Check sheet for the modelled part. Datum: model origin and axes. Units: mm. A direction names the side the tool comes from. Round coordinates to 2 decimals unless told otherwise and drop trailing zeros. Write each loop counter-clockwise with the first axis right and the second up, starting at its lowest first coordinate (ties: lowest second). Pieces come first, ordered by that corner, then holes. Notation, with made-up numbers: (66.5, 85.5) -> (109.5, 85.5) arc R20 cw to (109.5, 114.5) -> close; hole circle Ø8 at (35.5, 62.5). An arc over 180 degrees is marked (long way). Put each result on its own line as item: value. Start each with the question number.
Autodesk Inventor part; units mm, degrees
ref_plane "Work Plane2" through (-11, 0, 0) normal (1, 0, 0) x (0, 0, -1)
ref_plane "Work Plane3" through (0, 27, 0) normal (0, -1, 0) x (1, 0, 0)
ref_plane "YZ Plane" through (0, 0, 0) normal (1, 0, 0) x (0, 1, 0)
sketch "Sketch1" plane through (0, 0, 0) normal (0, 1, 0) x (-1, 0, 0)
  line L0 (0, 0) -> (22, 0)
  line L1 (22, 0) -> (22, -50)
  line L2 (22, -50) -> (0, -50)
  line L3 (0, -50) -> (0, 0)
  circle A0 centre (11, -8.5) radius 2.05
  circle A1 centre (11, -41.5) radius 2.05
  line L4 (22, 0) -> (0, -50) construction
  line L5 (22, -50) -> (0, 0) construction
  point P0 (11, -25)
  dimension "d0" = 22
  dimension "d1" = 50
  dimension "d2" = 4.1
  dimension "d3" = 4.1
  dimension "d5" = 33
  dimension "d40" = 16.5
extrude "Extrusion1" add sketch "Sketch1" along normal blind 5.5
sketch "Sketch3" plane through (0, 0, 0) normal (1, 0, 0) x (0, 0, -1)
  circle A0 centre (25, 16.3589) radius 6.4
  circle A1 centre (25, 16.3589) radius 14.4
  line L0 (50, 5.5) -> (0, 5.5)
  arc A2 (5.6002, 5.5) -> (11.0873, 12.6443) centre (5.6002, 11.1793) ccw
  arc A3 (38.9127, 12.6443) -> (44.3998, 5.5) centre (44.3998, 11.1793) ccw
  line L1 (0, 5.5) -> (50, 5.5)
  point P0 (0, 0)
  point P1 (25, 5.5)
  dimension "d11" = 12.8
  dimension "d12" = 8
extrude "Extrusion2" add sketch "Sketch3" against normal up to surface (22 mm away) contours A1 L0 | A1 L0 A2 | A3 L0 A1 picked at (24.7429, 7.0019)
sketch "Sketch4" plane through (0, 5.5, 0) normal (0, 1, 0) x (1, 0, 0)
  circle A0 centre (-11, 8.5) radius 2.05 construction
  circle A1 centre (-11, 8.5) radius 4.5
  circle A2 centre (-11, 41.5) radius 2.05 construction
  circle A3 centre (-11, 41.5) radius 4.5
  point P0 (0, 0)
  dimension "d15" = 9
  dimension "d16" = 9
extrude "Extrusion3" cut sketch "Sketch4" along normal through all
ref_plane "Work Plane2" through (-11, 0, 0) normal (1, 0, 0) x (0, 0, -1)
sketch "Sketch11" plane through (0, 0, 0) normal (1, 0, 0) x (0, 0, -1)
  line L0 (14.5852, 24.3188) -> (35.4148, 24.3188)
  line L1 (35.4148, 24.3188) -> (35.4148, 30.915)
  line L2 (30.4148, 35.915) -> (19.5852, 35.915)
  line L3 (14.5852, 30.915) -> (14.5852, 24.3188)
  line L4 (0, 0) -> (50, 0)
  arc A0 (19.5852, 35.915) -> (14.5852, 30.915) centre (19.5852, 30.915) ccw
  arc A1 (35.4148, 30.915) -> (30.4148, 35.915) centre (30.4148, 30.915) ccw
  point P0 (35.4148, 35.915)
  point P1 (14.5852, 35.915)
  point P2 (25, 24.3188)
  point P3 (25, 0)
  dimension "d49" = 5
extrude "Extrusion7" add sketch "Sketch11" against normal up to surface (22 mm away)
sketch "Sketch7" plane through (-11, 0, 0) normal (1, 0, 0) x (0, 0, -1)
  arc A0 (38.9127, 12.6443) -> (11.0873, 12.6443) centre (25, 16.3589) ccw construction
  line L0 (25, 16.3589) -> (25, 53.8517)
  line L1 (25, 40.4327) -> (28.1, 40.4327)
  line L2 (28.1, 40.4327) -> (28.1, 27.8589)
  line L3 (28.1, 27.8589) -> (28.1, 21.958)
  line L4 (28.1, 21.958) -> (25, 21.958)
  circle A1 centre (25, 16.3589) radius 6.4
  point P0 (0, 0)
  point P1 (25, 22.7589)
  point P2 (28.1, 30.4212)
  point P3 (25, 30.7589)
  dimension "d28" = 6.2
revolve "Revolution1" cut sketch "Sketch7" angle 360 about axis through (-11, 16.3589, -25) along (0, 1, 0) picked at (26.7389, 22.1049) contours L0 A1 L4 | L0 L1 L2 L3 A1
ref_plane "Work Plane3" through (0, 27, 0) normal (0, -1, 0) x (1, 0, 0)
sketch "Sketch10" plane through (0, 27, 0) normal (0, -1, 0) x (1, 0, 0)
  line L0 (-16.889, -25) -> (-13.9445, -19.9)
  line L1 (-13.9445, -19.9) -> (-8.0555, -19.9)
  line L2 (-8.0555, -19.9) -> (-5.111, -25) construction
  line L3 (-5.111, -25) -> (-8.0555, -30.1) construction
  line L4 (-8.0555, -30.1) -> (-13.9445, -30.1)
  line L5 (-13.9445, -30.1) -> (-16.889, -25)
  line L6 (-8.0555, -19.9) -> (0, -19.9)
  line L7 (0, -19.9) -> (0, -30.1)
  line L8 (0, -30.1) -> (-8.0555, -30.1)
  circle A0 centre (-11, -25) radius 3.1
  point P0 (0, 0)
  point P1 (-11, -21.9)
  dimension "d44" = 10.2
extrude "Extrusion6" cut sketch "Sketch10" along normal mid plane 5.2 contours L0 L1 L6 L7 L8 L4 L5 | A0
fillet "Fillet1" radius 5 2 edges at (-11, 26.3033, -35.4148) (-11, 26.3033, -14.5852)
chamfer "Chamfer1" distance 1 angle 45 22 edges at (-11, 5.5, 0) (-11, 5.5, -50) (0, 7.72, -10.1044) (0, 5.5, -2.8001) (0, 19.1603, -10.8751) (0, 19.1603, -39.1249) (0, 7.72, -39.8956) (0, 5.5, -47.1999) (-22, 19.1603, -39.1249) (-22, 7.72, -39.8956) (-22, 5.5, -47.1999) (-22, 19.1603, -10.8751) (-22, 7.72, -10.1044) (-22, 5.5, -2.8001) (-8.95, 5.5, -8.5) (-8.95, 5.5, -41.5) (0, 29.5264, -14.5852) (0, 29.5264, -35.4148) (0, 35.915, -25) (-22, 29.5264, -35.4148) (-22, 29.5264, -14.5852) (-22, 35.915, -25)
properties part number "narishige_holder"
1. Section check B-B, the plane z = -27. Enter the section's corners in (x, y) (3 decimals).
2. Gauge pin test, flat ends, axial feed: P1, Ø1, axis at x = -19.5, y = 15.5, coming from the -Z side; P2, Ø3, axis at x = -13.5, y = 29, coming from the -Z side; P3, Ø2, axis at x = -7, y = 29.5, coming from the +Z side. Record the tip position at first contact, or that the pin passes through.
3. Material ranges on L1, parallel to Y at x = -12.25, z = -21 (3 decimals); L2, parallel to X at y = 33, z = -25; L3, parallel to Y at x = -2, z = -29.5 (3 decimals), recorded low to high. Write a range as [from, to].
4. Section check A-A, the plane x = -16.25. Enter the section's corners in (y, z) (3 decimals).
5. Access from +Z, -Z, +X, -X, +Y, -Y to the whole of each face (thin tool, end or side, straight path). Record for faces 1 (the flat face through (-11, 30, -14.585)), 2 (the flat face through (-11, 30, -35.415)), 3 (the flat face through (-0.507, 29.507, -15.078)).
6. Draft check along Y on faces 4 (the flat face through (-22, 10, -19)), 5 (the flat face through (-15.44, 27.04, -22.49)), 6 (the flat face through (-0.5, 5, -2.8)). Enter one of: released by +Y, released by -Y, zero draft, split by the parting line, or undercut.
Reply:
1. outline: (-22, 0) -> (0, 0) -> (0, 10.279) -> (-22, 10.279) -> close; (-22, 22.438) -> (-13.369, 22.438) -> (-13.369, 24.4) -> (-15.734, 24.4) -> (-15.734, 29.6) -> (-13.369, 29.6) -> (-13.369, 35.915) -> (-21, 35.915) -> (-22, 34.915) -> close; (-8.631, 22.438) -> (0, 22.438) -> (0, 24.4) -> (-8.631, 24.4) -> close; (-8.631, 29.6) -> (0, 29.6) -> (0, 34.915) -> (-1, 35.915) -> (-8.631, 35.915) -> close
2. P1: stops at z = -39.4
2. P2: stops at z = -35.46
2. P3: stops at z = -14.59
3. L1: y = [0, 11.363], [21.355, 24.4], [29.6, 35.915]
3. L2: x = [-22, -14.1], [-7.9, 0]
3. L3: y = [0, 11.808], [20.91, 24.4], [29.6, 35.915]
4. outline: (0, -50) -> (4.5, -50) -> (5.5, -49) -> (5.5, -44.4) arc R5.679 cw to (12.644, -38.913) arc R14.4 ccw to (25.102, -36.442) arc R5 cw to (28.138, -35.415) -> (30.915, -35.415) arc R5 ccw to (35.915, -30.415) -> (35.915, -19.585) arc R5 ccw to (30.915, -14.585) -> (28.138, -14.585) arc R5 cw to (25.102, -13.558) arc R14.4 ccw to (12.644, -11.087) arc R5.679 cw to (5.5, -5.6) -> (5.5, -1) -> (4.5, 0) -> (0, 0) -> close; hole circle Ø12.8 at (16.359, -25); hole (24.4, -26.107) -> (29.6, -26.107) -> (29.6, -23.893) -> (24.4, -23.893) -> close
5. face 1: +Z, +X, -X, +Y
5. face 2: -Z, +X, -X, +Y
5. face 3: +Z, +X, +Y
6. face 4: zero draft
6. face 5: undercut
6. face 6: released by +Y
